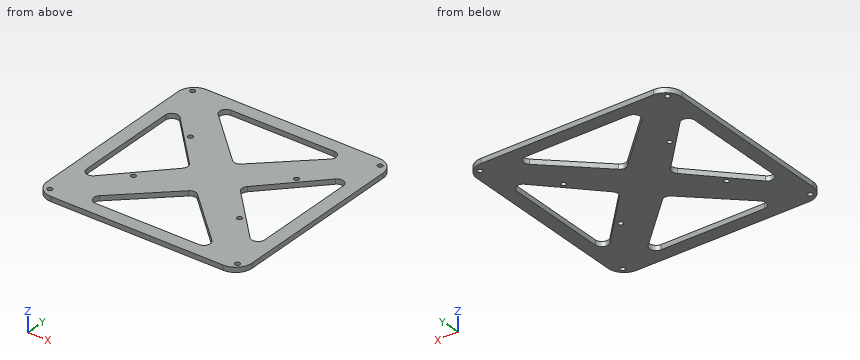
from build123d import *

# Parameters (mm, degrees)
SKETCH_1_W      = 125.6
SKETCH_1_H      = 125.3
SKETCH_1_R      = 1.5
EXTRUDE_1_DEPTH = 3
FILLET_1_R      = 10
FILLET_2_R      = 4


with BuildPart() as part:
    # 草图1 → 凸台-拉伸1 (new body)
    with BuildSketch(Plane.XY):
        with Locations((62.8, -62.65)):
            Rectangle(SKETCH_1_W, SKETCH_1_H)
        with Locations((30.3, -39.65)):
            Circle(SKETCH_1_R, mode=Mode.SUBTRACT)
        with Locations((95.3, -39.65)):
            Circle(SKETCH_1_R, mode=Mode.SUBTRACT)
        with Locations((95.3, -85.65)):
            Circle(SKETCH_1_R, mode=Mode.SUBTRACT)
        with Locations((30.3, -85.65)):
            Circle(SKETCH_1_R, mode=Mode.SUBTRACT)
        with Locations((120.3, -120.15)):
            Circle(SKETCH_1_R, mode=Mode.SUBTRACT)
        with Locations((5.3, -120.15)):
            Circle(SKETCH_1_R, mode=Mode.SUBTRACT)
        with Locations((5.3, -5.15)):
            Circle(SKETCH_1_R, mode=Mode.SUBTRACT)
        with Locations((120.3, -5.15)):
            Circle(SKETCH_1_R, mode=Mode.SUBTRACT)
        Polygon((21.089760081, -117.229442096), (104.510239919, -117.229442096), (62.8, -77.778125501), align=None, mode=Mode.SUBTRACT)
        Polygon((8.220557904, -104.360239919), (47.671874499, -62.65), (8.220557904, -20.939760081), align=None, mode=Mode.SUBTRACT)
        Polygon((21.089760081, -8.070557904), (62.8, -47.521874499), (104.510239919, -8.070557904), align=None, mode=Mode.SUBTRACT)
        Polygon((117.379442096, -20.939760081), (77.928125501, -62.65), (117.379442096, -104.360239919), align=None, mode=Mode.SUBTRACT)
    extrude(amount=EXTRUDE_1_DEPTH)

    # 圆角1
    fillet_1_edges = [part.edges().sort_by_distance(p)[0] for p in [
        (0, 0, 1.5),
        (125.6, 0, 1.5),
        (125.6, -125.3, 1.5),
        (0, -125.3, 1.5),
    ]]
    fillet(fillet_1_edges, radius=FILLET_1_R)

    # 圆角2
    fillet_2_edges = [part.edges().sort_by_distance(p)[0] for p in [
        (62.8, -77.778125501, 1.5),
        (21.089760081, -117.229442096, 1.5),
        (104.510239919, -117.229442096, 1.5),
        (47.671874499, -62.65, 1.5),
        (8.220557904, -20.939760081, 1.5),
        (8.220557904, -104.360239919, 1.5),
        (62.8, -47.521874499, 1.5),
        (104.510239919, -8.070557904, 1.5),
        (21.089760081, -8.070557904, 1.5),
        (77.928125501, -62.65, 1.5),
        (117.379442096, -104.360239919, 1.5),
        (117.379442096, -20.939760081, 1.5),
    ]]
    fillet(fillet_2_edges, radius=FILLET_2_R)


solid = part.part
Verification items for the finished model (mm, model axes). Give positions to 0.01 mm unless a question says otherwise; leave off trailing zeros. Write each loop counter-clockwise with the first axis right and the second up, starting at its lowest first coordinate (ties: lowest second). Pieces come first, ordered by that corner, then holes. Notation, with made-up numbers: M 8,-38.75 L 33,-38.75 A25 ccw 33,-3.75 Z; hole C 67.25,-8.75 d8. An arc over 180 degrees is marked long. Put each result on its own line as item: value. Start each with the question number.
1. Section check B-B (y = -120.15). Record the cut outline in (x, z), and give its area (3 significant figures).
2. Scan lines: line 1 along X through (y, z) = (-85.65, 2.1); line 2 along Y through (x, z) = (5.3, 0.7); line 3 along Y through (x, z) = (30.3, 0.65). Record each from-to range of solid material in increasing order. Write a range as [from, to].
3. Section check D-D (y = -85.65). Record the cut outline in (x, z).
4. Section check C-C (x = 120.3). Record the cut outline in (y, z).
5. Section check A-A (x = 92). Record the cut outline in (y, z), and give its area (3 significant figures).
Answer list:
1. outline: M 1.25,0 L 3.8,0 L 3.8,3 L 1.25,3 Z; M 6.8,0 L 118.8,0 L 118.8,3 L 6.8,3 Z; M 121.8,0 L 124.35,0 L 124.35,3 L 121.8,3 Z
1. area: 351 mm2
2. line 1: [0, 8.22], [25.92, 28.8], [31.8, 54.48], [71.12, 93.8], [96.8, 99.68], [117.38, 125.6]
2. line 2: [-124.13, -121.65], [-118.65, -6.65], [-3.65, -1.17]
2. line 3: [-125.3, -117.14], [-108.52, -87.15], [-84.15, -81.02], [-44.28, -41.15], [-38.15, -16.78], [-8.16, 0]
3. outline: M 0,0 L 8.22,0 L 8.22,3 L 0,3 Z; M 25.92,0 L 28.8,0 L 28.8,3 L 25.92,3 Z; M 31.8,0 L 54.48,0 L 54.48,3 L 31.8,3 Z; M 71.12,0 L 93.8,0 L 93.8,3 L 71.12,3 Z; M 96.8,0 L 99.68,0 L 99.68,3 L 96.8,3 Z; M 117.38,0 L 125.6,0 L 125.6,3 L 117.38,3 Z
4. outline: M -124.13,0 L -121.65,0 L -121.65,3 L -124.13,3 Z; M -118.65,0 L -6.65,0 L -6.65,3 L -118.65,3 Z; M -3.65,0 L -1.17,0 L -1.17,3 L -3.65,3 Z
5. outline: M -125.3,0 L -117.23,0 L -117.23,3 L -125.3,3 Z; M -105.4,0 L -77.53,0 L -77.53,3 L -105.4,3 Z; M -47.77,0 L -19.9,0 L -19.9,3 L -47.77,3 Z; M -8.07,0 L 0,0 L 0,3 L -8.07,3 Z
5. area: 216 mm2
